```python
from build123d import *

# Parameters (mm, degrees)
CYLINDER_W        = 15.5
CYLINDER_H        = 12
CYLINDER_ANGLE    = 180
CYLINDER001_W     = 15.5
CYLINDER001_H     = 12
CYLINDER001_ANGLE = 180
BOX_W             = 31
BOX_H             = 37
BOX_DEPTH         = 12
FILLET_R          = 2


with BuildPart() as obj1:
    # Cylinder → Cylinder (revolve)
    with BuildSketch(Plane.XZ.offset(-18.5)):
        with Locations((7.75, 6)):
            Rectangle(CYLINDER_W, CYLINDER_H)
    revolve(axis=Axis((0, 18.5, 0), (0, 0, 1)), revolution_arc=CYLINDER_ANGLE)


with BuildPart() as obj2:
    # Cylinder001 → Cylinder001 (revolve)
    with BuildSketch(Plane(origin=(0, -18.5, 0), x_dir=(-1, 0, 0), z_dir=(0, 1, 0))):
        with Locations((7.75, 6)):
            Rectangle(CYLINDER001_W, CYLINDER001_H)
    revolve(axis=Axis((0, -18.5, 0), (0, 0, 1)), revolution_arc=CYLINDER001_ANGLE)


with BuildPart() as obj3:
    # Box → Box (new body)
    with BuildSketch(Plane(origin=(-15.5, -18.5, 0), x_dir=(1, 0, 0), z_dir=(0, 0, 1))):
        with Locations((15.5, 18.5)):
            Rectangle(BOX_W, BOX_H)
    extrude(amount=BOX_DEPTH)

    # Fusion: union obj1, obj2
    add(obj1.part)
    add(obj2.part)

    # Fillet
    fillet_edges = [obj3.edges().sort_by_distance(p)[0] for p in [
        (-15.5, 0, 12),
    ]]
    fillet(fillet_edges, radius=FILLET_R)


with BuildPart() as obj3_1:
    # Fillet placement: moved
    add(obj3.part.moved(Location((0, 0, 40))))


solid = obj3_1.part
```
Build history of the part. All positions in model axes, mm. Coordinates: 2 decimals unless noted, no trailing zeros. Order: outer loops, then holes, each group sorted by start corner. A loop starts at its lowest first (then second) coordinate and runs counter-clockwise, first axis right, second up. Notation, with made-up numbers: (1, 72.25) -> (14, 72.25) arc R35 ccw to (14, 108.25) -> close; hole circle Ø1 at (88, -13). An arc over 180 degrees is marked (long way). Answer in a Markdown table with one row per item. Add a question column.
Q1. Band-saw the part on A-A, the plane z = 42.25. List the corners of the cut face in (x, y), then the cut area to 3 significant figures.
Q2. Drop a flat-ended pin along its axis: pin 1 (1 mm diameter, centred on x = -1.5, z = 50, fed in from +Y). Give the stop position or say it passes through.
Q3. Wall check: line 1 along Z through (x, y) = (7.5, 30); line 2 along Y through (x, z) = (0, 45.25); line 3 along Y through (x, z) = (-5, 49.25). Give the ranges that are in metal, low to high. Write a range as [from, to].
Answers follow:
| question | item | result |
|---|---|---|
| 1 | outline | (-15.5, -18.5) arc R15.5 ccw to (15.5, -18.5) -> (15.5, 18.5) arc R15.5 ccw to (-15.5, 18.5) -> close |
| 1 | area | 1,900 mm^2 |
| 2 | pin 1 | y = 33.97 |
| 3 | line 1 | [40, 51.99] |
| 3 | line 2 | [-34, 34] |
| 3 | line 3 | [-33.17, 33.17] |
